from build123d import *

# Parameters (mm, degrees)
F1_DEPTH = 25.6


with BuildPart() as f1:
    # F0 (on Top) → F1 (new body)
    with BuildSketch(Plane.XY):
        Polygon((56.2, 0), (0, 0), (0, -27.4), (3, -27.4), (3, -4.5), (3, -2.5), (5, -2.5), (51.7, -2.5), (53.7, -2.5), (53.7, -4.5), (53.7, -27.4), (56.2, -27.4), align=None)
        Polygon((51.7, -2.5), (53.7, -4.5), (53.7, -2.5), align=None)
        Polygon((3, -2.5), (3, -4.5), (5, -2.5), align=None)
    extrude(amount=F1_DEPTH)


solid = f1.part
Here's how the part is built. I have some questions about the finished solid (model axes, mm). A direction names the side the tool comes from. Round coordinates to 2 decimals unless told otherwise and drop trailing zeros. Order: outer loops, then holes, each group sorted by start corner. A loop starts at its lowest first (then second) coordinate and runs counter-clockwise, first axis right, second up. Notation, with made-up numbers: M 7.25,19 L 34.25,19 A21 ccw 34.25,27 Z; hole C 16.25,12.25 d6. An arc over 180 degrees is marked long. Return JSON: item names as keys, results as strings. Group by question number.
1. If we section it at A-A on y = -11.5: List the corners of the cut face in (x, z) for me.
2. If we mould it in two halves opening along X, with no side actions, what happens to faces 3 (the face through (52.7, -3.5, 12.6)), 4 (the face through (56.2, -14, 13)), 5 (the face through (55, -27.4, 13)), 6 (the face through (0, -14, 13))? For each: pulls with the +X half, pulls with the -X half, needs draft (parallel to the pull), parting line crosses it, or undercut.
3. I'm going to push a flat-ended pin straight in: pin 1 Ø6 at (x, z) = (43.5, 10.5) entering from -Y. Where does the tip first touch, or does it pass through?
4. On a 3-axis mill with a long thin cutter (end or side, diameter ignored), from which of +Z, -Z, +X, -X, +Y, -Y can I reach the whole of each face in a straight line? I mean faces 1 (the face through (4, -3.5, 12.6)), 2 (the face through (26, -2, 0)). Say none if no direction works.
5. If we section it at C-C on x = 30.5: List the corners of the cut face in (y, z) for me.
6. If we section it at B-B on z = 10: List the corners of the cut face in (x, y) for me.
7. Please list where these lines run through material, in increasing order: probe 1 along X at (y, z) = (-18.5, 16.25); probe 2 along Y at (x, z) = (50, 7); probe 3 along Y at (x, z) = (4, 18.75).
Reply:
{
 "1": {"outline": "M 0,0 L 3,0 L 3,25.6 L 0,25.6 Z; M 53.7,0 L 56.2,0 L 56.2,25.6 L 53.7,25.6 Z"},
 "2": {"face 3": "undercut", "face 4": "pulls with the +X half", "face 5": "needs draft", "face 6": "pulls with the -X half"},
 "3": {"pin 1": "y = -2.5"},
 "4": {"face 1": "+Z, -Z, -Y", "face 2": "-Z, +X, -X, +Y, -Y"},
 "5": {"outline": "M -2.5,0 L 0,0 L 0,25.6 L -2.5,25.6 Z"},
 "6": {"outline": "M 0,-27.4 L 3,-27.4 L 3,-4.5 L 5,-2.5 L 51.7,-2.5 L 53.7,-4.5 L 53.7,-27.4 L 56.2,-27.4 L 56.2,0 L 0,0 Z"},
 "7": {"probe 1": "0 to 3, 53.7 to 56.2", "probe 2": "-2.5 to 0", "probe 3": "-3.5 to 0"}
}
